from build123d import *

# Parameters (mm, degrees)
LINEAR_AUSTRAGEN_D_NN1_DEPTH    = 20
FASE1_SIZE                      = 3
SKIZZE2_R                       = 3.25
SCHNITT_LINEAR_AUSTRAGEN1_DEPTH = 10
SKIZZE3_R                       = 3.25
SCHNITT_LINEAR_AUSTRAGEN2_DEPTH = 10


with BuildPart() as part:
    # Skizze1 → Linear-Austragen-Dünn1 (new, symmetric)
    with BuildSketch(Plane.XY):
        Polygon((0, 20), (0, 0), (20, 0), (20, 1), (1, 1), (1, 20), align=None)
    extrude(amount=LINEAR_AUSTRAGEN_D_NN1_DEPTH, both=True)

    # Fase1
    fase1_edges = [part.edges().sort_by_distance(p)[0] for p in [
        (0.5, 20, 20),
        (0.5, 20, -20),
        (20, 0.5, -20),
        (20, 0.5, 20),
    ]]
    chamfer(fase1_edges, length=FASE1_SIZE)

    # Skizze2 → Schnitt-Linear austragen1 (cut)
    with BuildSketch(Plane(origin=(0, 1, 0), x_dir=(1, 0, 0), z_dir=(0, 1, 0))):
        with Locations(Location((10, -6, 0), (0, 0, 270))):
            Circle(SKIZZE2_R)
    extrude(amount=-SCHNITT_LINEAR_AUSTRAGEN1_DEPTH, mode=Mode.SUBTRACT)

    # Skizze3 → Schnitt-Linear austragen2 (cut)
    with BuildSketch(Plane(origin=(1, 0, 0), x_dir=(0, 0, -1), z_dir=(1, 0, 0))):
        with Locations(Location((14, 14, 0), (0, 0, 90))):
            Circle(SKIZZE3_R)
    extrude(amount=-SCHNITT_LINEAR_AUSTRAGEN2_DEPTH, mode=Mode.SUBTRACT)


solid = part.part
Could you check a few things on this model? Use its own coordinates, in mm. A direction names the side the tool comes from. Round coordinates to 2 decimals unless told otherwise and drop trailing zeros. Order: outer loops, then holes, each group sorted by start corner. A loop starts at its lowest first (then second) coordinate and runs counter-clockwise, first axis right, second up. Notation, with made-up numbers: M -13.5,-4 L 36.5,-4 A29 ccw 36.5,34 Z; hole C -1,65 d7. An arc over 180 degrees is marked long. One line per item, written item: value.
(1) If we mould it in two halves opening along Y, with no side actions, what happens to faces 1 (the cylindrical face through (0.507, 10.753, -13.857)), 2 (the flat face through (0, 10, 0)), 3 (the flat face through (10, 0, 0)), 4 (the flat face through (11, 1, 0))? For each: released by +Y, released by -Y, zero draft, split by the parting line, or undercut.
Ans:
face 1: undercut
face 2: zero draft
face 3: released by -Y
face 4: released by +Y
(2) I'm going to push flat-ended pins straight in: P1, Ø10.5, axis at y = 14, z = -14, coming from the +X side; P2, Ø1.5, axis at x = 17, z = -11.5, coming from the +Y side; P3, Ø5, axis at y = 7, z = -10, coming from the -X side; P4, Ø1.5, axis at x = 10.5, z = 4, coming from the +Y side. Where does each tip first touch, or does it pass through?
Ans:
P1: stops at x = 1
P2: stops at y = 1
P3: stops at x = 0
P4: passes through
(3) I need wall thicknesses on line 1 along Z through (x, y) = (0.5, 14); line 2 along X through (y, z) = (0.4, 6); line 3 along Y through (x, z) = (11.5, -18). Which ranges of each line are inside material? Lowest first, please. Write a range as from..to.
Ans:
line 1: z = -20..-17.25, -10.75..20
line 2: x = 0..6.75, 13.25..20
line 3: y = 0..1
(4) Imagine slicing it at D-D (x = 4). Write out the boundary of the cut face in (y, z).
Ans:
outline: M 0,-20 L 1,-20 L 1,20 L 0,20 Z
(5) Imagine slicing it at B-B (x = 10). Write out the boundary of the cut face in (y, z), and give its area (3 significant figures).
Ans:
outline: M 0,-20 L 1,-20 L 1,2.75 L 0,2.75 Z; M 0,9.25 L 1,9.25 L 1,20 L 0,20 Z
area: 33.5 mm^2
(6) Imagine slicing it at C-C (y = 14.75). Write out the boundary of the cut face in (x, z).
Ans:
outline: M 0,-20 L 1,-20 L 1,-17.16 L 0,-17.16 Z; M 0,-10.84 L 1,-10.84 L 1,20 L 0,20 Z
(7) Imagine slicing it at A-A (z = 6). Write out the boundary of the cut face in (x, y).
Ans:
outline: M 0,0 L 6.75,0 L 6.75,1 L 1,1 L 1,20 L 0,20 Z; M 13.25,0 L 20,0 L 20,1 L 13.25,1 Z
(8) Which directions (+Z, -Z, +X, -X, +Y, -Y) give clear straight access to the entire face, cutting with the end or side of a thin tool? Please do faces 5 (the flat face through (0.5, 20, 0.2)), 6 (the flat face through (1, 10, 0)).
Ans:
face 5: +Z, -Z, +X, -X, +Y
face 6: +Z, -Z, +X, +Y
